Could you check a few things on this model? Use its own coordinates, in mm. Face numbers are marked on the shaded views. A direction names the side the tool comes from. Give positions to 0.01 mm unless a question says otherwise; leave off trailing zeros. Write each loop counter-clockwise with the first axis right and the second up, starting at its lowest first coordinate (ties: lowest second). Pieces come first, ordered by that corner, then holes. Notation, with made-up numbers: (7, -5.5) -> (53, -5.5) arc R20 ccw to (53, 14.5) -> close; hole circle Ø11 at (-20.5, 76.25). An arc over 180 degrees is marked (long way). Write item = value, one per line. Start each with the question number.
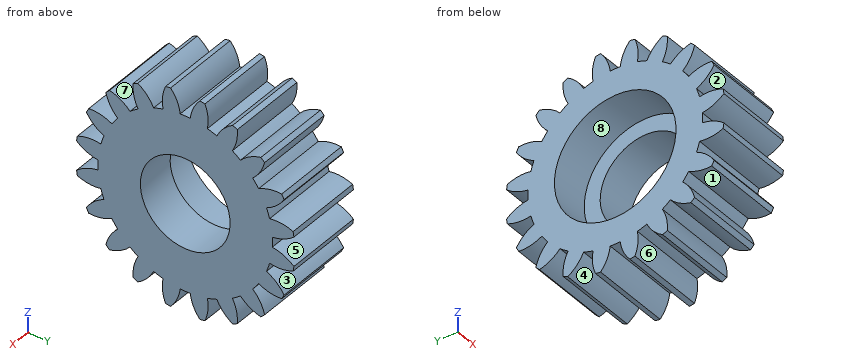
```python
from build123d import *

# Parameters (mm, degrees)
BASPROSKE_W        = 10
BASPROSKE_H        = 11
TOOTHCUT_DEPTH     = 19.493242009
TEETHCUTS_COUNT    = 20
TEETHCUTS_ANGLE    = 342
BORSKE_R           = 2.5
BORE_DEPTH         = 50.0000508
SKETCH1_R          = 6.1
CUT_EXTRUDE1_DEPTH = 4
SKETCH2_R          = 4.5
CUT_EXTRUDE2_DEPTH = 19.376827944
SKETCH3_R          = 14.898414192
CUT_EXTRUDE3_DEPTH = 2


with BuildPart() as part:
    # BasProSke → Base-Revolve (revolve)
    with BuildSketch(Plane(origin=(0, 0, 0), x_dir=(1, 0, 0), z_dir=(0, 1, 0)), mode=Mode.PRIVATE) as base_revolve_sk:
        with Locations((5, 5.5)):
            Rectangle(BASPROSKE_W, BASPROSKE_H)
    revolve(base_revolve_sk.sketch.rotate(Axis((-10, 0, 0), (1, 0, 0)), 180), axis=Axis((-10, 0, 0), (1, 0, 0)))

    # TooCutSke → ToothCut (cut, through all)
    with BuildSketch(Plane(origin=(0, 0, 0), x_dir=(0, 0, -1), z_dir=(1, 0, 0))):
        with BuildLine():
            ThreePointArc((0.499924007, 8.734705318), (0, 8.749), (-0.499924007, 8.734705318))
            ThreePointArc((-0.499924007, 8.734705318), (-0.824302243, 9.905497836), (-1.485192705, 10.924909509))
            ThreePointArc((-1.485192705, 10.924909509), (0, 11.0254), (1.485192705, 10.924909509))
            ThreePointArc((1.485192705, 10.924909509), (0.824302243, 9.905497836), (0.499924007, 8.734705318))
        make_face()
    toothcut = extrude(amount=TOOTHCUT_DEPTH, mode=Mode.SUBTRACT)

    # TeethCuts: ToothCut ×20 about axis
    teethcuts_axis = Axis((-10, 0, 0), (1, 0, 0))
    for i in range(1, TEETHCUTS_COUNT):
        add(toothcut.rotate(teethcuts_axis, i * TEETHCUTS_ANGLE / (TEETHCUTS_COUNT - 1)), mode=Mode.SUBTRACT)

    # BorSke → Bore (cut, symmetric)
    with BuildSketch(Plane(origin=(0, 0, 0), x_dir=(0, 0, -1), z_dir=(1, 0, 0))):
        with Locations(Location((0, 0, 0), (0, 0, 180))):
            Circle(BORSKE_R)
    extrude(amount=BORE_DEPTH, both=True, mode=Mode.SUBTRACT)

    # Sketch1 → Cut-Extrude1 (cut)
    with BuildSketch(Plane.ZY):
        Circle(SKETCH1_R)
    extrude(amount=-CUT_EXTRUDE1_DEPTH, mode=Mode.SUBTRACT)

    # Sketch2 → Cut-Extrude2 (cut, through all)
    with BuildSketch(Plane(origin=(10, 0, 0), x_dir=(0, 0, -1), z_dir=(1, 0, 0))):
        Circle(SKETCH2_R)
    extrude(amount=-CUT_EXTRUDE2_DEPTH, mode=Mode.SUBTRACT)

    # Sketch3 → Cut-Extrude3 (cut)
    with BuildSketch(Plane(origin=(10, 0, 0), x_dir=(0, 0, -1), z_dir=(1, 0, 0))):
        Circle(SKETCH3_R)
    extrude(amount=-CUT_EXTRUDE3_DEPTH, mode=Mode.SUBTRACT)


solid = part.part
```
(1) Imagine slicing it at A-A (z = 0). Please give me the cut outline in (x, y), then the cut area to 3 significant figures.
(2) I'm going to push flat-ended pins straight in: pin 1 (2 mm diameter, centred on y = -6, z = -2, fed in from -X); pin 2 (11 mm diameter, centred on y = 0, z = 0, fed in from -X). Where does each tip first touch, or does it pass through?
(3) If I drill on line 1 along Z through (x, y) = (0.75, -8.5); line 2 along Z through (x, y) = (1, -9); line 3 along Y through (x, z) = (6.6, 0), over which ranges is the centre line in solid material (lowest first)? Write a range as from..to.
(4) We'd pull the mould along Y, two halves only. Please class the marked faces 1, 2 and 3: released by +Y, released by -Y, zero draft, split by the parting line, or undercut.
(5) On a 3-axis mill with a long thin cutter (end or side, diameter ignored), from which of +Z, -Z, +X, -X, +Y, -Y can I reach the whole of each face in a straight line? I mean the marked faces 4, 5, 6, 7 and 8. Say none if no direction works.
Answers below:
q1.outline = (0, -8.75) -> (8, -8.75) -> (8, -4.5) -> (4, -4.5) -> (4, -6.1) -> (0, -6.1) -> close; (0, 6.1) -> (4, 6.1) -> (4, 4.5) -> (8, 4.5) -> (8, 8.75) -> (0, 8.75) -> close
q1.area = 55.2 mm^2
q2.pin_1 = 0
q2.pin_2 = 4
q3.line_1 = -5.16..-3.36, -2.23..2.23, 3.36..5.16
q3.line_2 = -5.23..-3.7, -2.29..-0.54, 0.54..2.29, 3.7..5.23
q3.line_3 = -8.75..-4.5, 4.5..8.75
q4.face_1 = undercut
q4.face_2 = released by -Y
q4.face_3 = released by +Y
q5.face_4 = -Z, +X, -X
q5.face_5 = +X, -X, +Y
q5.face_6 = +X, -X
q5.face_7 = +Z, +X, -X
q5.face_8 = -X
